Verification items for the finished model (mm, model axes). Face numbers are marked on the shaded views. A direction names the side the tool comes from. Round coordinates to 2 decimals unless told otherwise and drop trailing zeros. Order: outer loops, then holes, each group sorted by start corner. A loop starts at its lowest first (then second) coordinate and runs counter-clockwise, first axis right, second up.
```python
from build123d import *

# Parameters (mm, degrees)
BOSS_EXTRUDE1_DEPTH      = 300
BOSS_EXTRUDE1_DEPTH_BACK = 50
F_3_0_3_DIAMETER_HOLE3_D = 3
F_3_0_3_DIAMETER_HOLE4_D = 3


with BuildPart() as part:
    # Sketch1 → Boss-Extrude1 (new, two sides: drawn at the far end of the back side and taken through both)
    with BuildSketch(Plane(origin=(0, 0, 0), x_dir=(1, 0, 0), z_dir=(0, 1, 0)).offset(-BOSS_EXTRUDE1_DEPTH_BACK)):
        Polygon((0, 0), (0, 10), (2, 10), (2, 2), (20, 2), (20, 0), align=None)
    extrude(amount=BOSS_EXTRUDE1_DEPTH + BOSS_EXTRUDE1_DEPTH_BACK)

    # Ø3.0 (3) Diameter Hole3 (through all)
    with Locations(Plane(origin=(2, 311.407632793, -241.32004832), x_dir=(0, 0, 1), z_dir=(1, 0, 0))):
        with Locations((235.32004832, 355.407632793), (235.32004832, 341.407632793)):
            Hole(F_3_0_3_DIAMETER_HOLE3_D / 2)

    # Ø3.0 (3) Diameter Hole4 (through all)
    with Locations(Plane(origin=(2, 311.407632793, -241.32004832), x_dir=(0, 0, 1), z_dir=(1, 0, 0))):
        with Locations((235.32004832, 17.407632793), (235.32004832, 31.407632793)):
            Hole(F_3_0_3_DIAMETER_HOLE4_D / 2)


solid = part.part
```
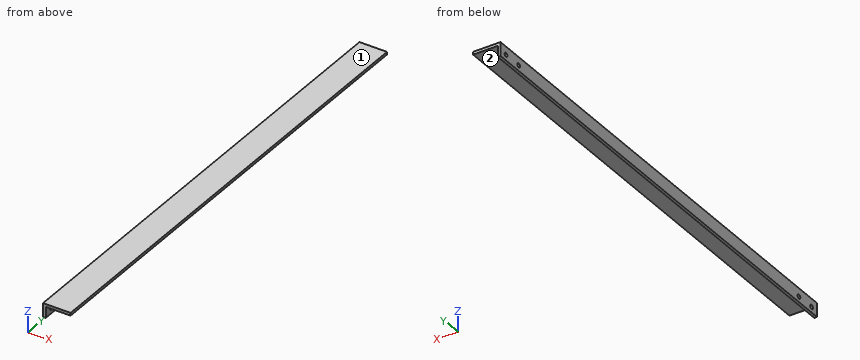
1) Tool access check on the marked faces 1 and 2. Record the directions out of +Z, -Z, +X, -X, +Y, -Y that give a thin tool (end or side, any length) a straight path to the whole face; none if there is none.
2) Scan lines: probe 1 along Y at (x, z) = (1.1, -6); probe 2 along Z at (x, y) = (0.65, 280); probe 3 along Z at (x, y) = (3.75, 206). Record each from-to range of solid material in increasing order.
3) Sectioned sample at C-C on x = 10.75. Record the cut outline in (y, z), then the cut area to 3 significant figures.
4) Sectioned sample at B-B on y = 104. Record the cut outline in (x, z).
5) Go/stop test with flat-tipped pins: pin 1 Ø10 at (x, y) = (10.5, 195.5) entering from -Z; pin 2 Ø4 at (x, y) = (16.5, 140.5) entering from +Z; pin 3 Ø5 at (y, z) = (280, -6) entering from +X. Record where each tip stops, or that it passes through.
6) Sectioned sample at A-A on z = -6. Record the cut outline in (x, y).
Returned:
1. face 1: +Z, +X, -X, +Y, -Y
1. face 2: -Z, +X, +Y, -Y
2. probe 1: y = -50 to -45.5, -42.5 to -31.5, -28.5 to 278.5, 281.5 to 292.5, 295.5 to 300
2. probe 2: z = -10 to -7.5, -4.5 to 0
2. probe 3: z = -2 to 0
3. outline: (-50, -2) - (300, -2) - (300, 0) - (-50, 0) - close
3. area: 700 mm2
4. outline: (0, -10) - (2, -10) - (2, -2) - (20, -2) - (20, 0) - (0, 0) - close
5. pin 1: stops at z = -2
5. pin 2: stops at z = 0
5. pin 3: stops at x = 2
6. outline: (0, -50) - (2, -50) - (2, -45.5) - (0, -45.5) - close; (0, -42.5) - (2, -42.5) - (2, -31.5) - (0, -31.5) - close; (0, -28.5) - (2, -28.5) - (2, 278.5) - (0, 278.5) - close; (0, 281.5) - (2, 281.5) - (2, 292.5) - (0, 292.5) - close; (0, 295.5) - (2, 295.5) - (2, 300) - (0, 300) - close
